Autodesk Inventor part; units mm, degrees
ref_plane "Work Plane1" through (0, 1.5, 0) normal (0, -1, 0) x (1, 0, 0)
ref_plane "YZ Plane" through (0, 0, 0) normal (1, 0, 0) x (0, 1, 0)
ref_plane "XZ Plane" through (0, 0, 0) normal (0, 1, 0) x (-1, 0, 0)
sketch "Sketch1" plane through (0, 0, 0) normal (0, 1, 0) x (-1, 0, 0)
  line L0 (-8.55, 0) -> (-8.55, 0)
  line L1 (5.4, 2.35) -> (-5.4, 2.35)
  line L2 (-7.75, 0) -> (-7.75, 0)
  line L3 (7.75, 0) -> (7.75, 0)
  arc A0 (-5.4, 2.35) -> (-7.75, 0) centre (-5.4, 0) ccw
  arc A1 (-7.75, 0) -> (-5.4, -2.35) centre (-5.4, 0) ccw
  arc A2 (7.75, 0) -> (5.4, 2.35) centre (5.4, 0) ccw
  arc A3 (5.4, -2.35) -> (7.75, 0) centre (5.4, 0) ccw
  circle A4 centre (5.4, 0) radius 1.5
  circle A5 centre (-5.4, 0) radius 1.5
  circle A6 centre (2.3, 0) radius 0.75
  circle A7 centre (0, 0) radius 0.75
  circle A8 centre (-2.3, 0) radius 0.75
  circle A9 centre (2.3, 0) radius 0.35
  circle A10 centre (0, 0) radius 0.35
  circle A11 centre (-2.3, 0) radius 0.45
  line L4 (-15.2366, 19.4813) -> (26.8433, 19.4813) construction
  line L5 (26.8433, 19.4813) -> (26.8433, -5.0467) construction
  line L6 (26.8433, -5.0467) -> (-15.2366, -5.0467) construction
  line L7 (-15.2366, -5.0467) -> (-15.2366, 19.4813) construction
  line L8 (-8.3717, -2.35) -> (8.3717, -2.35)
  line L9 (8.3717, 2.35) -> (-8.3717, 2.35)
  circle A12 centre (2.3, 0) radius 1.05
  circle A13 centre (0, 0) radius 1.05
  circle A14 centre (-2.3, 0) radius 1.05
  point P0 (7.75, 0)
  point P1 (-5.4, -2.35)
  point P2 (5.4, -2.35)
  dimension "d5" = 2.35
  dimension "d6" = 3
  dimension "d7" = 3
  dimension "d10" = 1.5
  dimension "d11" = 4.6
  dimension "d14" = 0.9
  dimension "d201" = 2.1
  dimension "d202" = 2.1
  dimension "d203" = 2.1
  dimension "d204" = 1.5
  dimension "d205" = 1.5
extrude "Extrusion1" add sketch "Sketch1" along normal blind 6 contours A2 A3 L8 A1 A0 L1 | A12 | A13 | A14
ref_plane "Work Plane1" through (0, 1.5, 0) normal (0, -1, 0) x (1, 0, 0)
sketch "Sketch2" plane through (0, 1.5, 0) normal (0, -1, 0) x (1, 0, 0)
  line L0 (0, 0) -> (9.8, 0)
  circle A0 centre (9.8, 0) radius 1
  circle A1 centre (9.8, 0) radius 1.85
  circle A2 centre (9.8, 0) radius 2.75
  line L1 (-8.3604, 2.3431) -> (8.3604, 2.3431)
  line L2 (8.3604, -2.3431) -> (-8.3604, -2.3431)
  line L3 (-8.1293, 2.1844) -> (8.1293, -2.1844) construction
  line L4 (8.1293, 2.1844) -> (-8.7202, -2.3431) construction
  line L5 (0, 0) -> (-9.8, 0)
  circle A3 centre (-9.8, 0) radius 1
  circle A4 centre (-9.8, 0) radius 1.85
  circle A5 centre (-9.8, 0) radius 2.75
  dimension "d119" = 9.8
  dimension "d120" = 2
  dimension "d121" = 3.7
  dimension "d122" = 5.5
  dimension "d126" = 9.8
  dimension "d127" = 2
  dimension "d128" = 3.7
  dimension "d130" = 5.5
extrude "Extrusion2" add sketch "Sketch2" against normal blind 2 contours L5 A5 L1 A2 L0 | L0 A2 L2 A5 L5
extrude "Extrusion3" add sketch "Sketch2" against normal blind 2 contours A2 | A5
extrude "Extrusion4" add sketch "Sketch2" against normal blind 1.2 contours A1 | A3 | A4
sketch "Sketch3" plane through (-5.4, 0, 2.35) normal (0, 0, 1) x (1, 0, 0)
  line L0 (-9.7661, 9.6728) -> (32.2033, 9.6728) construction
  line L1 (32.2033, 9.6728) -> (32.2033, -14.7908) construction
  line L2 (32.2033, -14.7908) -> (-9.7661, -14.7908) construction
  line L3 (-9.7661, -14.7908) -> (-9.7661, 9.6728) construction
  point P0 (5.4, 0)
extrude "Extrusion5" cut sketch "Sketch2" against normal through all contours A0 | A3
extrude "Extrusion6" cut sketch "Sketch1" along normal through all contours A4 | A5
extrude "Extrusion7" cut sketch "Sketch1" along normal blind 10 contours A6 | A7 | A8 | A9 | A10 | A11
extrude "Extrusion8" cut sketch "Sketch1" along normal blind 0.5 contours A12 | A13 | A14
properties part number "Pogo2" material "Nylon 6/6"
Model file for the job. Use its own axes, mm. A direction names the side the tool comes from. Give positions to 0.01 mm unless a question says otherwise; leave off trailing zeros. Loops run counter-clockwise (first coordinate to the right, second up) from the corner with the lowest first, then second, coordinate; pieces in that order, holes last. Notation, with made-up numbers: M 36,40 L 47,40 A31 cw 47,67 Z; hole C 58,-21 d6. An arc over 180 degrees is marked long. Use one line per item in the form item = value.
Item 1: Slice it at C-C on y = 2.4. List the corners of the cut face in (x, z).
Filled in:
outline = M -8.36,-2.34 L -5.58,-2.34 A2.35 ccw -5.4,-2.35 L 5.4,-2.35 A2.35 ccw 5.58,-2.34 L 8.36,-2.34 A2.75 ccw long 8.36,2.34 L 5.58,2.34 A2.35 ccw 5.4,2.35 L -5.4,2.35 A2.35 ccw -5.58,2.34 L -8.36,2.34 A2.75 ccw long Z; hole C -9.8,0 d2; hole C -5.4,0 d3; hole C -2.3,0 d1.5; hole C 0,0 d1.5; hole C 2.3,0 d1.5; hole C 5.4,0 d3; hole C 9.8,0 d2
Item 2: Two-plate mould, pull along X, no slides. Class faces 5 (the flat face through (8, 3.5, -1)), 6 (the flat face through (11, 2.7, -1)): released by +X, released by -X, zero draft, split by the parting line, or undercut.
Filled in:
face_5 = zero draft
face_6 = undercut
Item 3: Slice it at A-A on y = 5.45. List the corners of the cut face in (x, z), and give its area (3 significant figures).
Filled in:
outline = M -5.4,-2.35 L 5.4,-2.35 A2.35 ccw 5.4,2.35 L -5.4,2.35 A2.35 ccw Z; hole C -5.4,0 d3; hole C -2.3,0 d1.5; hole C 0,0 d1.5; hole C 2.3,0 d1.5; hole C 5.4,0 d3
area = 48.7 mm^2
Item 4: Flat gauge pins, fed straight in: pin 1 Ø1.6 at (x, y) = (-7, 3) entering from +Z; pin 2 Ø3 at (x, z) = (10, 1) entering from +Y; pin 3 Ø2 at (y, z) = (5.5, -1) entering from +X. Where does each tip first touch, or does it go through?
Filled in:
pin_1 = 2.34
pin_2 = 3.5
pin_3 = 7.75
Item 5: Which spindle directions (+Z, -Z, +X, -X, +Y, -Y) get a long thin tool onto all of the face, cutting with end or side? Do faces 1 (the cylindrical face through (-12.55, 2.49, 0.08)), 2 (the flat face through (-7, 2, 2.343)), 3 (the flat face through (0, 3, -2.35)), 4 (the flat face through (-9, 2.7, -1)). Say none if no direction does.
Filled in:
face_1 = +Y, -Y
face_2 = +Z, +Y, -Y
face_3 = -Z, +Y, -Y
face_4 = +Y
Item 6: Slice it at B-B on x = -9.8. List the corners of the cut face in (y, z), and give its area (3 significant figures).
Filled in:
outline = M 1.5,-2.75 L 3.5,-2.75 L 3.5,-1.85 L 2.7,-1.85 L 2.7,-1 L 1.5,-1 Z; M 1.5,1 L 2.7,1 L 2.7,1.85 L 3.5,1.85 L 3.5,2.75 L 1.5,2.75 Z
area = 5.64 mm^2
Item 7: Slice it at D-D on z = 0. Give the number of separate pieces and of enclosed holes in the cut face, and give its area (3 significant figures).
Filled in:
separate_pieces = 8
enclosed_holes = 0
area = 37.6 mm^2
Item 8: Drill centre lines: L1, parallel to Z at x = 2.3, y = 2.8; L2, parallel to X at y = 4.2, z = 0.8; L3, parallel to Z at x = -9.8, y = 3.35. Where is each one in solid material? Low to high.
Filled in:
L1 = -2.35 to -0.75, 0.75 to 2.35
L2 = -7.61 to -6.67, -4.13 to 4.13, 6.67 to 7.61
L3 = -2.75 to -1.85, 1.85 to 2.75
